```python
from build123d import *

# Parameters (mm, degrees)
EXTRUDE_1_DEPTH      = 6
SKETCH_2_R           = 2.55
CUT_EXTRUDE_1_DEPTH  = 7
SKETCH_21_W          = 7
SKETCH_21_H          = 6
EXTRUDE_2_DEPTH      = 6
CUT_EXTRUDE_11_DEPTH = 7
SKETCH_22_W          = 7
SKETCH_22_H          = 6
EXTRUDE_21_DEPTH     = 6
SKETCH_24_W          = 7
SKETCH_24_H          = 6
EXTRUDE_23_DEPTH     = 6
CUT_EXTRUDE_14_DEPTH = 7
SKETCH_25_W          = 7
SKETCH_25_H          = 6
EXTRUDE_24_DEPTH     = 6
SKETCH_26_W          = 7
SKETCH_26_H          = 6
EXTRUDE_25_DEPTH     = 6
SKETCH_27_W          = 7
SKETCH_27_H          = 6
EXTRUDE_26_DEPTH     = 6
SKETCH_28_W          = 7
SKETCH_28_H          = 6
EXTRUDE_27_DEPTH     = 6
SKETCH_29_W          = 7
SKETCH_29_H          = 6
EXTRUDE_28_DEPTH     = 6


with BuildPart() as part:
    # Эскиз1 → Бобышка-Вытянуть1 (new body)
    with BuildSketch(Plane(origin=(0, 0, 0), x_dir=(1, 0, 0), z_dir=(0, 1, 0))):
        with BuildLine():
            Line((-35, -65), (-35, -75))
            Line((-35, -75), (-25, -75))
            ThreePointArc((-25, -75), (-17.928932188, -72.071067812), (-15, -65))
            ThreePointArc((-15, -65), (-2.368853025, -29.632779179), (29.809139443, -10.26881824))
            ThreePointArc((29.809139443, -10.26881824), (40.031565804, -0.046391879), (29.809139443, 10.176034483))
            ThreePointArc((29.809139443, 10.176034483), (-2.372594749, 29.596870998), (-15, 65))
            ThreePointArc((-15, 65), (-17.928932188, 72.071067812), (-25, 75))
            Line((-25, 75), (-35, 75))
            Line((-35, 75), (-35, 65))
            Line((-35, 65), (-35, -65))
        make_face()
    extrude(amount=EXTRUDE_1_DEPTH)

    # Эскиз2 → Вырез-Вытянуть1 (cut, through all)
    with BuildSketch(Plane.XZ):
        with Locations((-25, -65)):
            Circle(SKETCH_2_R)
        with Locations((-25, 65)):
            Circle(SKETCH_2_R)
        with BuildLine():
            Line((28, -2.55), (25.5, -2.55))
            ThreePointArc((25.5, -2.55), (22.95, 0), (25.5, 2.55))
            Line((25.5, 2.55), (28, 2.55))
            ThreePointArc((28, 2.55), (30.55, 0), (28, -2.55))
        make_face()
    extrude(amount=-CUT_EXTRUDE_1_DEPTH, mode=Mode.SUBTRACT)

    # Эскиз21 → Бобышка-Вытянуть2 (add)
    with BuildSketch(Plane(origin=(15, 6, -43.5), x_dir=(0, 0, -1), z_dir=(0, 1, 0))):
        with Locations((-9.531849908, 53)):
            Rectangle(SKETCH_21_W, SKETCH_21_H)
        with Locations((9.531849908, 53)):
            Rectangle(SKETCH_21_W, SKETCH_21_H)
    extrude(amount=-EXTRUDE_2_DEPTH)

    # Эскиз31 → Вырез-Вытянуть11 (cut, through all)
    with BuildSketch(Plane(origin=(15, 6, -43.5), x_dir=(0, 0, -1), z_dir=(0, 1, 0))):
        Polygon((-2.1, 45), (-3.6, 45), (-3.6, 42.6), (-2.1, 42.6), (-2.1, 39), (2.1, 39), (2.1, 42.6), (3.6, 42.6), (3.6, 45), (2.1, 45), (2.1, 50), (-2.1, 50), align=None)
    extrude(amount=-CUT_EXTRUDE_11_DEPTH, mode=Mode.SUBTRACT)

    # Эскиз22 → Бобышка-Вытянуть21 (add)
    with BuildSketch(Plane(origin=(15, 0, -43.5), x_dir=(0, 0, 1), z_dir=(0, -1, 0))):
        with Locations((-9.531849908, 53)):
            Rectangle(SKETCH_22_W, SKETCH_22_H)
        with Locations((9.531849908, 53)):
            Rectangle(SKETCH_22_W, SKETCH_22_H)
    extrude(amount=-EXTRUDE_21_DEPTH)

    # Эскиз24 → Бобышка-Вытянуть23 (add)
    with BuildSketch(Plane(origin=(15, 0, 43.5), x_dir=(0, 0, 1), z_dir=(0, -1, 0))):
        with Locations((-9.531849908, 53)):
            Rectangle(SKETCH_24_W, SKETCH_24_H)
        with Locations((9.531849908, 53)):
            Rectangle(SKETCH_24_W, SKETCH_24_H)
    extrude(amount=-EXTRUDE_23_DEPTH)

    # Эскиз34 → Вырез-Вытянуть14 (cut, through all)
    with BuildSketch(Plane(origin=(15, 0, 43.5), x_dir=(0, 0, 1), z_dir=(0, -1, 0))):
        Polygon((-2.1, 45), (-3.6, 45), (-3.6, 42.6), (-2.1, 42.6), (-2.1, 39), (2.1, 39), (2.1, 42.6), (3.6, 42.6), (3.6, 45), (2.1, 45), (2.1, 50), (-2.1, 50), align=None)
    extrude(amount=-CUT_EXTRUDE_14_DEPTH, mode=Mode.SUBTRACT)

    # Эскиз25 → Бобышка-Вытянуть24 (add)
    with BuildSketch(Plane(origin=(15, 6, 43.5), x_dir=(0, 0, -1), z_dir=(0, 1, 0))):
        with Locations((-9.531849908, 53)):
            Rectangle(SKETCH_25_W, SKETCH_25_H)
        with Locations((9.531849908, 53)):
            Rectangle(SKETCH_25_W, SKETCH_25_H)
    extrude(amount=-EXTRUDE_24_DEPTH)

    # Эскиз26 → Бобышка-Вытянуть25 (add)
    with BuildSketch(Plane(origin=(15, 6, -43.5), x_dir=(0, 0, -1), z_dir=(0, 1, 0))):
        with Locations((-9.531849908, 53)):
            Rectangle(SKETCH_26_W, SKETCH_26_H)
        with Locations((9.531849908, 53)):
            Rectangle(SKETCH_26_W, SKETCH_26_H)
    extrude(amount=-EXTRUDE_25_DEPTH)

    # Эскиз27 → Бобышка-Вытянуть26 (add)
    with BuildSketch(Plane(origin=(15, 6, 43.5), x_dir=(0, 0, -1), z_dir=(0, 1, 0))):
        with Locations((-9.531849908, 53)):
            Rectangle(SKETCH_27_W, SKETCH_27_H)
        with Locations((9.531849908, 53)):
            Rectangle(SKETCH_27_W, SKETCH_27_H)
    extrude(amount=-EXTRUDE_26_DEPTH)

    # Эскиз28 → Бобышка-Вытянуть27 (add)
    with BuildSketch(Plane(origin=(15, 0, -43.5), x_dir=(0, 0, 1), z_dir=(0, -1, 0))):
        with Locations((-9.531849908, 53)):
            Rectangle(SKETCH_28_W, SKETCH_28_H)
        with Locations((9.531849908, 53)):
            Rectangle(SKETCH_28_W, SKETCH_28_H)
    extrude(amount=-EXTRUDE_27_DEPTH)

    # Эскиз29 → Бобышка-Вытянуть28 (add)
    with BuildSketch(Plane(origin=(15, 0, 43.5), x_dir=(0, 0, 1), z_dir=(0, -1, 0))):
        with Locations((-9.531849908, 53)):
            Rectangle(SKETCH_29_W, SKETCH_29_H)
        with Locations((9.531849908, 53)):
            Rectangle(SKETCH_29_W, SKETCH_29_H)
    extrude(amount=-EXTRUDE_28_DEPTH)


solid = part.part
```
For this review, take the finished solid that the model builds, in its own axes (mm). A direction names the side the tool comes from. Give positions to 0.01 mm unless a question says otherwise; leave off trailing zeros. Write each loop counter-clockwise with the first axis right and the second up, starting at its lowest first coordinate (ties: lowest second). Pieces come first, ordered by that corner, then holes. Notation, with made-up numbers: M 65,-36.5 L 106,-36.5 A25 ccw 106,-6.5 Z; hole C 3.25,-37 d3. An arc over 180 degrees is marked long. Answer as CSV lines item,"result".
1. Draft analysis for pull direction Z (two halves, no side actions). For faces 4 (the flat face through (-33, 3, -41.4)), 5 (the flat face through (-38, 3, 56.532)), 6 (the cylindrical face through (40.03, 2.96, 0.27)), state which applies: +Z half, -Z half, draft (parallel to the pull), parting line (faces both ways), or undercut.
Findings:
face 4,"undercut"
face 5,"+Z half"
face 6,"parting line"
2. For faces 1 (the flat face through (-35, 3, 48)), 2 (the flat face through (-38, 3, -56.532)), 3 (the cylindrical face through (22.95, 2.96, -0.06)), list the 3-axis set-ups (+Z, -Z, +X, -X, +Y, -Y) from which the entire face can be reached by the end or side of a thin tool; tool diameter is ignored.
Findings:
face 1,"-X, +Y, -Y"
face 2,"-Z, -X, +Y, -Y"
face 3,"+Y, -Y"
3. Consider section B-B, the plane z = 0. Write out the cut boundary in (x, y), then the cut area to 3 significant figures.
Findings:
outline,"M -35,0 L 22.95,0 L 22.95,6 L -35,6 Z; M 30.55,0 L 40.03,0 L 40.03,6 L 30.55,6 Z"
area,"405 mm2"
4. Consider section D-D, the plane x = -5. Write out the cut boundary in (y, z), then the cut area to 3 significant figures.
Findings:
outline,"M 0,-33.08 L 6,-33.08 L 6,33.12 L 0,33.12 Z"
area,"397 mm2"
5. Consider section C-C, the plane y = 1. Count the separate pieces of the cut face and the enclosed holes in it, then the cut area to 3 significant figures.
Findings:
separate pieces,"1"
enclosed holes,"3"
area,"5,260 mm2"
6. Consider section A-A, the plane x = -33.5. Write out the cut boundary in (y, z), then the cut area to 3 significant figures.
Findings:
outline,"M 0,-75 L 6,-75 L 6,-45.6 L 0,-45.6 Z; M 0,-41.4 L 6,-41.4 L 6,41.4 L 0,41.4 Z; M 0,45.6 L 6,45.6 L 6,75 L 0,75 Z"
area,"850 mm2"
7. For pin 1 (2 mm diameter, centred on y = 4.5, z = 44.5, fed in from -X); pin 2 (1.2 mm diameter, centred on y = 3, z = -41, fed in from -X); pin 3 (3 mm diameter, centred on x = -19.5, y = 3.5, fed in from -Z), all flat-tipped, find the tip position at first contact; note any pin that passes through.
Findings:
pin 1,"stops at x = -24"
pin 2,"stops at x = -35"
pin 3,"stops at z = -74.17"
8. Wall thickness on line 1 (Z direction, x = -25, y = 2); line 2 (Z direction, x = -30.5, y = 0.7); line 3 (Z direction, x = 24, y = 3.1): over which ranges is each line inside the solid? List them lowest first.
Findings:
line 1,"z = -75 to -67.55, -62.45 to -45.6, -41.4 to 41.4, 45.6 to 62.45, 67.55 to 75"
line 2,"z = -75 to -45.6, -41.4 to 41.4, 45.6 to 75"
line 3,"z = -11.68 to -2.06, 2.06 to 11.77"
